For this review, take the finished solid that the model builds, in its own axes (mm). A direction names the side the tool comes from. Give positions to 0.01 mm unless a question says otherwise; leave off trailing zeros. Order: outer loops, then holes, each group sorted by start corner. A loop starts at its lowest first (then second) coordinate and runs counter-clockwise, first axis right, second up.
Autodesk Fusion 360 part; units mm, degrees
sketch "Sketch1" plane through (0, 0, 0) normal (0, 1, 0) x (1, 0, 0)
  circle A0 centre (30, 0) radius 5
  line L0 (33.328, 9.43) -> (6.6508, 18.845)
  line L1 (33.328, -9.43) -> (6.6508, -18.845)
  arc A1 (33.328, -9.43) -> (33.328, 9.43) centre (30, 0) ccw
  arc A2 (6.6508, 18.845) -> (6.6508, -18.845) centre (0, 0) ccw
  line L2 (-2.25, 2.3452) -> (-2.25, -2.3452)
  arc A3 (-2.25, -2.3452) -> (-2.25, 2.3452) centre (0, 0) ccw
extrude "Extrude1" add sketch "Sketch1" along normal blind 4 contours A0 | L0 L1 A1 A2
extrude "Extrude2" add sketch "Sketch1" against normal blind 35 contours A0
1) Tool access review of faces 5 (the face through (3.25, 1.97, -0.11)), 6 (the face through (25, -17, 0)): name each direction out of +Z, -Z, +X, -X, +Y, -Y from which nothing blocks a thin tool from reaching the whole face with its end or side.
Answer sheet:
face 5: +Y, -Y
face 6: -Y
2) To check wall thickness, follow line 1 (Z direction, x = 0, y = 1); line 2 (Y direction, x = 14, z = -5.5); line 3 (X direction, y = 0.5, z = -2). State the ranges of each line that lie inside material, in increasing order.
Answer sheet:
line 1: z = -19.98 to -3.25, 3.25 to 19.98
line 2: y = 0 to 4
line 3: x = -19.88 to -2.25, 2.56 to 39.8
3) We need section B-B on z = 0. Give the boundary of the cut face in (x, y), then the cut area to 3 significant figures.
Answer sheet:
outline: (-19.98, 0) - (-2.25, 0) - (-2.25, 4) - (-19.98, 4) - close; (3.25, 0) - (25, 0) - (25, -35) - (35, -35) - (35, 0) - (40, 0) - (40, 4) - (3.25, 4) - close
area: 568 mm2
4) We need section A-A on x = 0. Give the boundary of the cut face in (y, z).
Answer sheet:
outline: (0, -19.98) - (4, -19.98) - (4, -3.25) - (0, -3.25) - close; (0, 3.25) - (4, 3.25) - (4, 19.98) - (0, 19.98) - close
5) Draft analysis for pull direction X (two halves, no side actions). For faces 1 (the face through (20.18, 1.97, 14.07)), 2 (the face through (-2.25, 2, 0)), 3 (the face through (10, 0, 0)), 4 (the face through (-19.977, 1.972, 0.534)), state which applies: +X half, -X half, draft (parallel to the pull), parting line (faces both ways), or undercut.
Answer sheet:
face 1: +X half
face 2: undercut
face 3: draft
face 4: parting line
6) Clearance check with flat-ended pins moving along their axes: pin 1 (4.5 mm diameter, centred on y = 2.5, z = -1, fed in from +X); pin 2 (1.5 mm diameter, centred on y = -1, z = -8, fed in from -X); pin 3 (7.5 mm diameter, centred on x = 0, z = 0, fed in from -Y); pin 4 (12 mm diameter, centred on y = -16, z = 2, fed in from +X). State where each tip first meets the part, or that it passes through.
Answer sheet:
pin 1: stops at x = 40
pin 2: passes through
pin 3: stops at y = 0
pin 4: stops at x = 35
7) We need section C-C on x = 30. Give the boundary of the cut face in (y, z), then the cut area to 3 significant figures.
Answer sheet:
outline: (-35, -5) - (0, -5) - (0, -10.6) - (4, -10.6) - (4, 10.6) - (0, 10.6) - (0, 5) - (-35, 5) - close
area: 435 mm2
8) We need section D-D on y = -4. Give the boundary of the cut face in (x, z).
Answer sheet:
outline: circle Ø10 at (30, 0)
